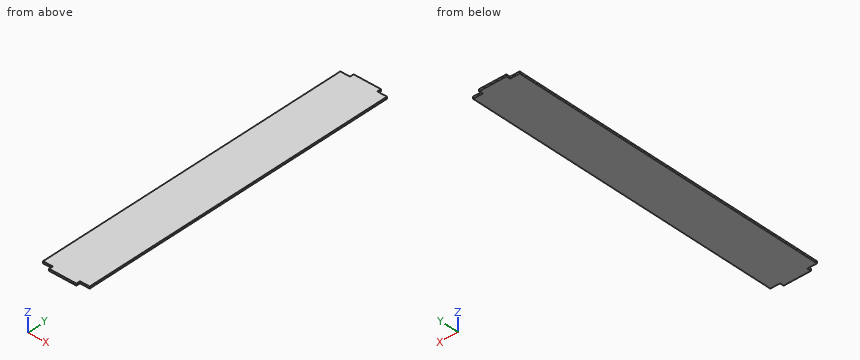
from build123d import *

# Parameters (mm, degrees)
F1_DEPTH = 425
F2_W     = 25
F2_H     = 10
F3_DEPTH = 5.001


with BuildPart() as f1:
    # F0 (on Front) → F1 (new body, symmetric)
    with BuildSketch(Plane.XZ):
        Polygon((-60, 5), (-60, 0), (0, 0), (60, 0), (60, 5), (0, 5), align=None)
    extrude(amount=F1_DEPTH, both=True)

    # F2 (on face) → F3 (cut, through all)
    with BuildSketch(Plane.XY.offset(5)):
        with Locations((47.5, -420)):
            Rectangle(F2_W, F2_H)
        with Locations((-47.5, -420)):
            Rectangle(F2_W, F2_H)
        with Locations((-47.5, 420)):
            Rectangle(F2_W, F2_H)
        with Locations((47.5, 420)):
            Rectangle(F2_W, F2_H)
    extrude(amount=-F3_DEPTH, mode=Mode.SUBTRACT)


solid = f1.part
The listing builds one solid part. Answer for the finished solid, in the listing's coordinates (mm). Round coordinates to 2 decimals unless told otherwise and drop trailing zeros. Order: outer loops, then holes, each group sorted by start corner. A loop starts at its lowest first (then second) coordinate and runs counter-clockwise, first axis right, second up. Notation, with made-up numbers: (61, 76.25) -> (81, 76.25) arc R36 ccw to (81, 115.25) -> close; hole circle Ø7 at (-34, -17.5). An arc over 180 degrees is marked (long way). One line per item, written item: value.
Item 1: A straight line is drawn through the part: L1, parallel to Y at x = 51, z = 3.55. Find the intervals that lie inside material, in ascending order.
Taken from the geometry:
L1: y = -415 to 415
Item 2: Given P1, Ø1.5, axis at x = 51.5, z = 3.5, coming from the -Y side; P2, Ø1.5, axis at y = -418.5, z = 3.5, coming from the +X side; P3, Ø6, axis at x = -26, y = 149.5, coming from the -Z side, each flat-ended and moving along its own axis, determine where each tip first touches the part or whether it passes through.
Taken from the geometry:
P1: stops at y = -415
P2: stops at x = 35
P3: stops at z = 0
Item 3: Find section A-A, the plane x = 51.5. Give the vertices of the cut face in (y, z), then the cut area to 3 significant figures.
Taken from the geometry:
outline: (-415, 0) -> (415, 0) -> (415, 5) -> (-415, 5) -> close
area: 4,150 mm2
